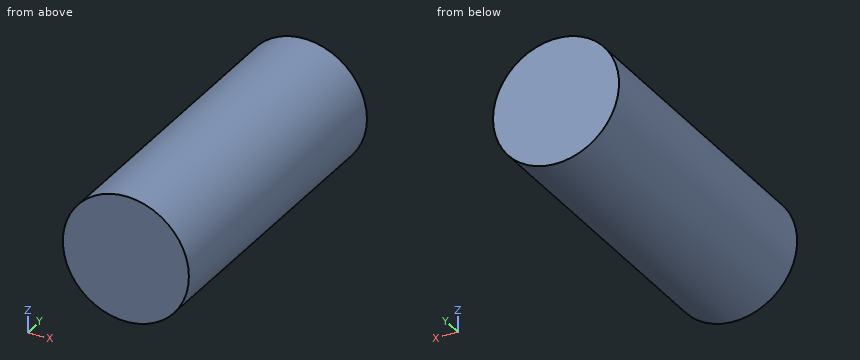
from build123d import *

# Parameters (mm, degrees)
F0_R     = 15
F1_DEPTH = 25
F2_DEPTH = 25
F3_DEPTH = 25


with BuildPart() as f1:
    # F0 (on Front) → F1 (new body)
    with BuildSketch(Plane.XZ):
        Circle(F0_R)
    extrude(amount=F1_DEPTH)

    # F2 (add): a face of the model
    f2_faces = [f1.faces().sort_by_distance(p)[0] for p in [
        (0, -25, 0),
    ]]
    extrude(f2_faces, amount=F2_DEPTH)

    # F3 (add): a face of the model
    f3_faces = [f1.faces().sort_by_distance(p)[0] for p in [
        (0, -50, 0),
    ]]
    extrude(f3_faces, amount=F3_DEPTH)


solid = f1.part
Build history of the part. All positions in model axes, mm. Round coordinates to 2 decimals unless told otherwise and drop trailing zeros. Loops run counter-clockwise (first coordinate to the right, second up) from the corner with the lowest first, then second, coordinate; pieces in that order, holes last. Notation, with made-up numbers: (21, 27) -> (71, 27) arc R25 ccw to (71, 46) -> close; hole circle Ø3 at (-24.5, -7.75). An arc over 180 degrees is marked (long way). Answer in a Markdown table with one row per item.
Item 1: Saw through at B-B (z = -6.5). Write the cut outline in (x, y).
Answers below:
| item | result |
|---|---|
| outline | (-13.52, -75) -> (13.52, -75) -> (13.52, 0) -> (-13.52, 0) -> close |
Item 2: Saw through at C-C (x = -3). Write the cut outline in (y, z).
Answers below:
| item | result |
|---|---|
| outline | (-75, -14.7) -> (0, -14.7) -> (0, 14.7) -> (-75, 14.7) -> close |
Item 3: Saw through at A-A (y = -47). Write the cut outline in (x, z).
Answers below:
| item | result |
|---|---|
| outline | circle Ø30 at (0, 0) |
Item 4: Drill centre lines: L1, parallel to Z at x = 5, y = -48; L2, parallel to X at y = -40.5, z = 2.75; L3, parallel to X at y = -56.5, z = -6.5. Where is each one in solid material? Low to high. Write a range as [from, to].
Answers below:
| item | result |
|---|---|
| L1 | z = [-14.14, 14.14] |
| L2 | x = [-14.75, 14.75] |
| L3 | x = [-13.52, 13.52] |
Item 5: Pin check, flat tips, straight feed: pin 1 (8 mm diameter, centred on x = 11, y = -54, fed in from -Z); pin 2 (5 mm diameter, centred on x = 4, y = -39, fed in from -Z); pin 3 (12 mm diameter, centred on x = 9.5, z = 2.5, fed in from +Y); pin 4 (3 mm diameter, centred on y = -8, z = -11.5, fed in from -X). Stop position of each tip, or through.
Answers below:
| item | result |
|---|---|
| pin 1 | stops at z = -13.27 |
| pin 2 | stops at z = -14.92 |
| pin 3 | stops at y = 0 |
| pin 4 | stops at x = -11.18 |
